The listing builds one solid part. Answer for the finished solid, in the listing's coordinates (mm). Coordinates: 2 decimals unless noted, no trailing zeros. Order: outer loops, then holes, each group sorted by start corner. A loop starts at its lowest first (then second) coordinate and runs counter-clockwise, first axis right, second up. Notation, with made-up numbers: M -27.5,-4 L -10.5,-4 A19 ccw -10.5,13 Z; hole C 38,-20.75 d1. An arc over 180 degrees is marked long. One line per item, written item: value. Start each with the question number.
Q1. The part is cut by section C-C on y = -15. Give the vertices of the cut face in (x, z), then the cut area to 3 significant figures.
Q2. The part is cut by section B-B on y = 18.5. Give the vertices of the cut face in (x, z), then the cut area to 3 significant figures.
Q3. This flat-tipped pin is pushed along its axis until it touches: pin 1 Ø1.9 at (x, y) = (-149.13, -22.5) entering from +Z. Where does it stop, or does it pass through?
Q4. The part is cut by section A-A on z = 2.35. Give the number of separate pieces and of enclosed holes in the cut face, then the cut area to 3 significant figures.
Q5. Straight lines are drawn through the part: line 1 along X through (y, z) = (-1, 3.05); line 2 along Y through (x, z) = (-22.5, 3.4); line 3 along Y through (x, z) = (22.5, 3.1). For each, find the intervals that lie inside material, in ascending order. Write a range as [from, to].
```python
from build123d import *

# Parameters (mm, degrees)
SKETCH2_R           = 1.5635
BOSS_EXTRUDE1_DEPTH = 5


with BuildPart() as part:
    # Sketch2 → Boss-Extrude1 (new body)
    with BuildSketch(Plane.XY):
        with BuildLine():
            Line((0, 27.5), (-229.132053392, 27.5))
            Line((-229.132053392, 27.5), (-229.132053392, -27.5))
            Line((-229.132053392, -27.5), (0, -27.5))
            ThreePointArc((0, -27.5), (27.5, 0), (0, 27.5))
        make_face()
        with Locations((0, 22.5)):
            Circle(SKETCH2_R, mode=Mode.SUBTRACT)
        with Locations((22.5, 0)):
            Circle(SKETCH2_R, mode=Mode.SUBTRACT)
        with Locations((0, -22.5)):
            Circle(SKETCH2_R, mode=Mode.SUBTRACT)
        with Locations((-22.5, 0)):
            Circle(SKETCH2_R, mode=Mode.SUBTRACT)
        with Locations((-171.632053392, 0)):
            Circle(SKETCH2_R, mode=Mode.SUBTRACT)
        with Locations((-149.132053392, 22.5)):
            Circle(SKETCH2_R, mode=Mode.SUBTRACT)
        with Locations((-126.632053392, 0)):
            Circle(SKETCH2_R, mode=Mode.SUBTRACT)
        with Locations((-149.132053392, -22.5)):
            Circle(SKETCH2_R, mode=Mode.SUBTRACT)
    extrude(amount=BOSS_EXTRUDE1_DEPTH)


solid = part.part
```
Output:
1. outline: M -229.13,0 L 23.05,0 L 23.05,5 L -229.13,5 Z
1. area: 1,260 mm^2
2. outline: M -229.13,0 L 20.35,0 L 20.35,5 L -229.13,5 Z
2. area: 1,250 mm^2
3. pin 1: passes through
4. separate pieces: 1
4. enclosed holes: 8
4. area: 13,700 mm^2
5. line 1: x = [-229.13, -172.83], [-170.43, -127.83], [-125.43, -23.7], [-21.3, 21.3], [23.7, 27.48]
5. line 2: y = [-27.5, -1.56], [1.56, 27.5]
5. line 3: y = [-15.81, -1.56], [1.56, 15.81]
